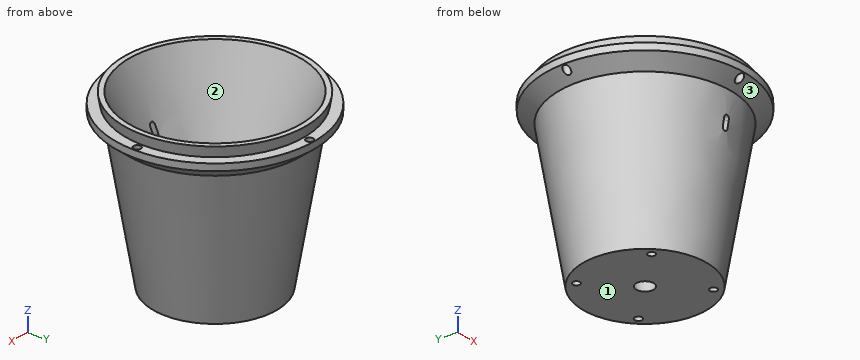
```python
from build123d import *

# Parameters (mm, degrees)
PAD_DEPTH       = 50
SKETCH_R        = 2.112176
SKETCH_R_2      = 2.082394
SKETCH_R_3      = 2.112641
SKETCH_R_4      = 2.091899
POCKET001_DEPTH = 12
SKETCH005_R     = 2.149119
SKETCH005_R_2   = 2.108774
SKETCH005_R_3   = 2.065142
SKETCH005_R_4   = 2.149709
POCKET002_DEPTH = 15


with BuildPart() as pad:
    # Sketch004 → Pad (new body)
    with BuildSketch(Plane.XZ):
        with BuildLine():
            ThreePointArc((1.645506, 70), (0, 71.645506), (-1.645506, 70))
            Line((-1.645506, 70), (-1.645506, 65.439445))
            ThreePointArc((-1.645506, 65.439445), (0, 63.793939), (1.645506, 65.439445))
            Line((1.645506, 70), (1.645506, 65.439445))
        make_face()
    extrude(amount=PAD_DEPTH)


with BuildPart() as obj1:
    # Sketch003 → Revolution001 (revolve)
    with BuildSketch(Plane.XZ):
        Polygon((5, 0), (50, 100), (53, 100), (52, 94), (58, 94), (58, 90), (50, 83.40284), (36, 0), align=None)
    revolve(axis=Axis((0, 0, 0), (0, 0, 1)))

    # Sketch → Pocket001 (cut)
    with BuildSketch(Plane(origin=(0, 0, 0), x_dir=(1, 0, 0), z_dir=(0, 0, -1))):
        with Locations((22, 22)):
            Circle(SKETCH_R)
        with Locations((-22, 22)):
            Circle(SKETCH_R_2)
        with Locations((22, -22)):
            Circle(SKETCH_R_3)
        with Locations((-22, -22)):
            Circle(SKETCH_R_4)
    extrude(amount=-POCKET001_DEPTH, mode=Mode.SUBTRACT)

    # Cut: cut Pad
    add(pad.part, mode=Mode.SUBTRACT)

    # Sketch005 → Pocket002 (cut)
    with BuildSketch(Plane.XY.offset(94)):
        with Locations((55.218414, -0.064825)):
            Circle(SKETCH005_R)
        with Locations((0, 55.39975)):
            Circle(SKETCH005_R_2)
        with Locations((-55.548775, 0)):
            Circle(SKETCH005_R_3)
        with Locations((0, -55.311054)):
            Circle(SKETCH005_R_4)
    extrude(amount=-POCKET002_DEPTH, mode=Mode.SUBTRACT)


solid = obj1.part
```
Input: part model. Units: mm. Frame: model coordinates. Face numbers are marked on the shaded views. Round coordinates to 2 decimals unless told otherwise and drop trailing zeros. Loops run counter-clockwise (first coordinate to the right, second up) from the corner with the lowest first, then second, coordinate; pieces in that order, holes last. Notation, with made-up numbers: (65, 21) -> (74, 21) arc R28 cw to (74, 39) -> close; hole circle Ø5 at (63.5, 58.5). An arc over 180 degrees is marked (long way). Use one line per item in the form item = value. Start each with the question number.
Item 1: Material intervals for L1, parallel to Y at x = -22, z = 6; L2, parallel to Y at x = -22, z = 3; L3, parallel to X at y = 22, z = 4.5, sorted ascending. Write a range as from..to.
Item 2: Contact query for flat-ended pins moving along their axis: pin 1 Ø8 at (x, y) = (-23, -14.5) entering from +Z; pin 2 Ø1 at (y, z) = (26.5, 25.5) entering from -X; pin 3 Ø3.5 at (y, z) = (-44, 67) entering from -X. Output: stop coordinate, or through.
Item 3: Section query B-B on z = 78. Return the cut outline in (x, y).
Item 4: Section query A-A on z = 14. Return the cut outline in (x, y).
Item 5: Mould query, pull axis Y, two halves, no side actions, for the marked faces 1, 2 and 3. Classes: pulls with the +Y half, pulls with the -Y half, needs draft (parallel to the pull), parting line crosses it, or undercut.
Ans:
q1.L1 = -29.76..-24.08, -19.92..19.91, 24.09..29.76
q1.L2 = -29.13..-24.08, -19.92..19.91, 24.09..29.13
q1.L3 = -29.44..-24.09, -19.91..19.89, 24.11..29.44
q2.pin_1 = 58.2
q2.pin_2 = -30.78
q2.pin_3 = -21.21
q3.outline = circle Ø98.19 at (0, 0); hole circle Ø80.2 at (0, 0)
q4.outline = circle Ø76.7 at (0, 0); hole circle Ø22.6 at (0, 0)
q5.face_1 = needs draft
q5.face_2 = undercut
q5.face_3 = parting line crosses it
